from build123d import *

# Parameters (mm, degrees)
F1_DEPTH      = 50.8
F1_DEPTH_BACK = 50.8


with BuildPart() as f1:
    # F0 (on Front) → F1 (new body, two sides)
    with BuildSketch(Plane.XZ) as f1_sk:
        with BuildLine():
            ThreePointArc((0, 0), (-28.342106, 32.569547), (-69.85, 44.45))
            Line((-69.85, 44.45), (-69.85, 0))
            Line((-69.85, 0), (-69.85, -44.45))
            Line((-69.85, -44.45), (0, -44.45))
            Line((0, -44.45), (69.85, -44.45))
            Line((69.85, -44.45), (69.85, -19.05))
            Line((69.85, -19.05), (44.45, -19.05))
            ThreePointArc((44.45, -19.05), (20.26992, -14.086852), (0, 0))
        make_face()
    extrude(amount=F1_DEPTH)
    extrude(f1_sk.sketch, amount=-F1_DEPTH_BACK)


solid = f1.part
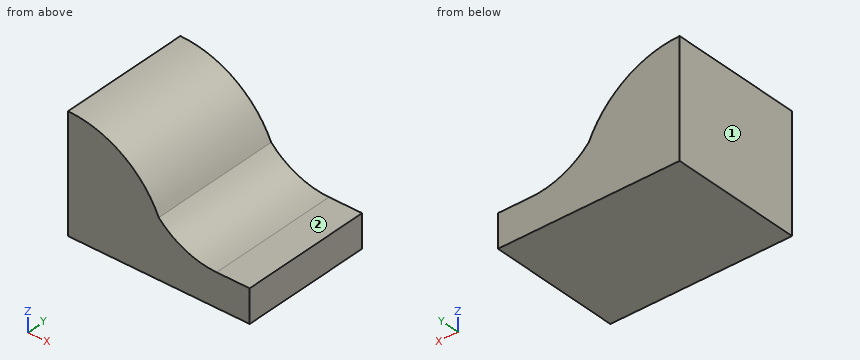
The listing builds one solid part. Answer for the finished solid, in the listing's coordinates (mm). Face numbers are marked on the shaded views. A direction names the side the tool comes from. Coordinates: 2 decimals unless noted, no trailing zeros. Loops run counter-clockwise (first coordinate to the right, second up) from the corner with the lowest first, then second, coordinate; pieces in that order, holes last.
1) Find section B-B on z = 27. Write down the section's boundary in (x, y), then the cut area to 3 significant figures.
2) Find section C-C on x = 14. Write down the section's boundary in (y, z).
3) A tool of negligible diameter and unlimited length cuts with its end or side. For the marked faces 1 and 2, from which of +Z, -Z, +X, -X, +Y, -Y can it reach the whole face along a straight path? Write none if from no direction.
4) Flat-ended cylindrical pins translate along their axes: pin 1 Ø6 at (x, y) = (25, 31.5) entering from +Z; pin 2 Ø7.5 at (x, y) = (54, -17) entering from +Z. Find the tip coordinate at first contact, or state that the pin passes through.
5) Find section A-A on y = -28. Write down the section's boundary in (x, z), then the cut area to 3 significant figures.
6) Find the intervals of material crossed by L1, parallel to Z at x = 63.5, y = 12; L2, parallel to Z at x = 26.5, y = 7; L3, parallel to X at y = -20, z = 32, in increasing order.
Values:
1. outline: (-69.85, -50.8) - (-20.69, -50.8) - (-20.69, 50.8) - (-69.85, 50.8) - close
1. area: 4,990 mm2
2. outline: (-50.8, -44.45) - (50.8, -44.45) - (50.8, -10.96) - (-50.8, -10.96) - close
3. face 1: +Z, -Z, -X, +Y, -Y
3. face 2: +Z, +X, +Y, -Y
4. pin 1: stops at z = -14.8
4. pin 2: stops at z = -19.05
5. outline: (-69.85, -44.45) - (69.85, -44.45) - (69.85, -19.05) - (44.45, -19.05) arc R61.38 cw to (0, 0) arc R76.01 ccw to (-69.85, 44.45) - close
5. area: 7,380 mm2
6. L1: z = -44.45 to -19.05
6. L2: z = -44.45 to -16.37
6. L3: x = -69.85 to -27.46
